```python
from build123d import *

# Parameters (mm, degrees)
F0_W     = 98.194085
F0_H     = 25.737483
F1_DEPTH = 5
F2_R     = 10
F3_R     = 10
F4_R     = 10
F6_DEPTH = 5.001


with BuildPart() as f1:
    # F0 (on Front) → F1 (new body)
    with BuildSketch(Plane.XZ):
        with Locations((14.827024, 13.008618)):
            Rectangle(F0_W, F0_H)
    extrude(amount=F1_DEPTH)

    # F2
    f2_edges = [f1.edges().sort_by_distance(p)[0] for p in [
        (63.924067, -2.5, 25.87736),
    ]]
    fillet(f2_edges, radius=F2_R)

    # F3
    f3_edges = [f1.edges().sort_by_distance(p)[0] for p in [
        (63.924067, -2.5, 0.139877),
    ]]
    fillet(f3_edges, radius=F3_R)

    # F4
    f4_edges = [f1.edges().sort_by_distance(p)[0] for p in [
        (-34.270018, -2.5, 25.87736),
    ]]
    fillet(f4_edges, radius=F4_R)

    # F5 (on face) → F6 (cut, through all)
    with BuildSketch(Plane.XZ.offset(5)):
        with BuildLine():
            ThreePointArc((-10.681925, 2.385375), (-5.498517, 2.031488), (-2.799221, 6.470717))
            ThreePointArc((-2.799221, 6.470717), (-5.581242, 10.951852), (-10.831449, 10.446342))
            ThreePointArc((-10.831449, 10.446342), (-12.782642, 6.877549), (-11.436118, 3.039539))
            Line((-11.436118, 3.039539), (-10.681925, 2.385375))
        make_face()
    extrude(amount=-F6_DEPTH, mode=Mode.SUBTRACT)


solid = f1.part
```
Build history of the part. All positions in model axes, mm. Round coordinates to 2 decimals unless told otherwise and drop trailing zeros. Write each loop counter-clockwise with the first axis right and the second up, starting at its lowest first coordinate (ties: lowest second). Pieces come first, ordered by that corner, then holes.
1) Band-saw the part on A-A, the plane z = 8.5. List the corners of the cut face in (x, y), and give its area (3 significant figures).
2) Band-saw the part on B-B, the plane y = -1.5. List the corners of the cut face in (x, z).
3) Drill centre lines: probe 1 along Z at (x, y) = (-8, -3.55); probe 2 along Z at (x, y) = (-10.5, -2); probe 3 along X at (y, z) = (-4.55, 10). Where is each one in solid material? Low to high.
4) Band-saw the part on D-D, the plane z = 24.5. List the corners of the cut face in (x, y).
5) Band-saw the part on C-C, the plane x = -8.5. List the corners of the cut face in (y, z).
Ans:
1. outline: (-34.27, -5) - (-12.37, -5) - (-12.37, 0) - (-34.27, 0) - close; (-3.23, -5) - (63.79, -5) - (63.79, 0) - (-3.23, 0) - close
1. area: 445 mm2
2. outline: (-34.27, 0.14) - (53.92, 0.14) arc R10 ccw to (63.92, 10.14) - (63.92, 15.88) arc R10 ccw to (53.92, 25.88) - (-24.27, 25.88) arc R10 ccw to (-34.27, 15.88) - close; hole (-11.44, 3.04) - (-10.68, 2.39) arc R5 ccw to (-2.8, 6.47) arc R5 ccw to (-10.83, 10.45) arc R5 ccw to start
3. probe 1: z = 0.14 to 1.47, 11.47 to 25.88
3. probe 2: z = 0.14 to 2.26, 10.68 to 25.88
3. probe 3: x = -34.27 to -11.34, -4.26 to 63.92
4. outline: (-29.33, -5) - (58.99, -5) - (58.99, 0) - (-29.33, 0) - close
5. outline: (-5, 0.14) - (0, 0.14) - (0, 1.52) - (-5, 1.52) - close; (-5, 11.42) - (0, 11.42) - (0, 25.88) - (-5, 25.88) - close
